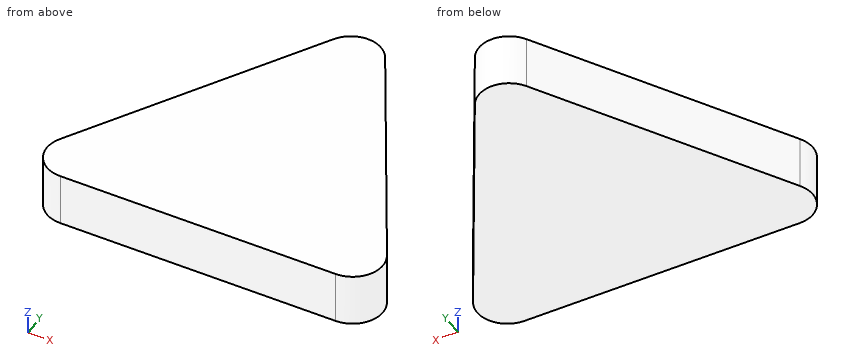
from build123d import *

# Parameters (mm, degrees)
BOSS_EXTRU_1_DEPTH = 3.5
CONG_1_R           = 2


with BuildPart() as part:
    # Esquisse1 → Boss.-Extru.1 (new body)
    with BuildSketch(Plane.XY):
        Polygon((-12.7, 0), (12.7, 0), (0, 21.997045256), align=None)
    extrude(amount=BOSS_EXTRU_1_DEPTH)

    # Congé1
    cong_1_edges = [part.edges().sort_by_distance(p)[0] for p in [
        (0, 21.997045256, 1.75),
        (12.7, 0, 1.75),
        (-12.7, 0, 1.75),
    ]]
    fillet(cong_1_edges, radius=CONG_1_R)


solid = part.part
Can you work these out from the model? Positions are in its coordinate system, mm. Coordinates: 2 decimals unless noted, no trailing zeros. Loops run counter-clockwise (first coordinate to the right, second up) from the corner with the lowest first, then second, coordinate; pieces in that order, holes last. Notation, with made-up numbers: (-27, 65.5) - (16, 65.5) arc R29 ccw to (16, 93.5) - close; hole circle Ø8 at (-18, 11.25). An arc over 180 degrees is marked (long way). Answer as a JSON object with one key per item and string values. Group by question number.
Item 1: If we section it at C-C (x = -8.75): List the corners of the cut face in (y, z) for me.
Item 2: If I drill on L1, parallel to X at y = 12.75, z = 1.2; L2, parallel to X at y = 2.5, z = 0.75; L3, parallel to Y at x = 10.25, z = 0.4, over which ranges is the centre line in solid material (lowest first)? Write a range as from..to.
Item 3: If we section it at B-B (y = 6): List the corners of the cut face in (x, z) for me, plus the area to 3 significant figures.
Item 4: For pin 1 (2 mm diameter, centred on y = 14, z = 2, fed in from +X), with a flat end and sliding along its axis, tell me the tip position at first contact or that it passes through.
Item 5: If we section it at A-A (z = 1.5): List the corners of the cut face in (x, y) for me.
Returned:
{
 "1": {"outline": "(0, 0) - (6.84, 0) - (6.84, 3.5) - (0, 3.5) - close"},
 "2": {"L1": "x = -5.34..5.34", "L2": "x = -11.17..11.17", "L3": "y = 0.28..4.24"},
 "3": {"outline": "(-9.24, 0) - (9.24, 0) - (9.24, 3.5) - (-9.24, 3.5) - close", "area": "64.7 mm²"},
 "4": {"pin 1": "stops at x = 5.19"},
 "5": {"outline": "(-10.97, 3) arc R2 ccw to (-9.24, 0) - (9.24, 0) arc R2 ccw to (10.97, 3) - (1.73, 19) arc R2 ccw to (-1.73, 19) - close"}
}
